```python
from build123d import *

# Parameters (mm, degrees)
SKETCH2_R           = 12.5
BOSS_EXTRUDE1_DEPTH = 6
SKETCH6_R           = 1.5
CUT_EXTRUDE1_DEPTH  = 15
SKETCH8_R           = 12.5
SKETCH8_R_2         = 10
BOSS_EXTRUDE2_DEPTH = 2
SKETCH9_R           = 2.5
CUT_EXTRUDE3_DEPTH  = 4


with BuildPart() as part:
    # Sketch2 → Boss-Extrude1 (new body)
    with BuildSketch(Plane.XY):
        Circle(SKETCH2_R)
    extrude(amount=BOSS_EXTRUDE1_DEPTH)

    # Sketch6 → Cut-Extrude1 (cut)
    with BuildSketch(Plane(origin=(0, 0, 0), x_dir=(-1, 0, 0), z_dir=(0, 0, -1))):
        with Locations((-5.488160471, -3.482828541)):
            Circle(SKETCH6_R)
        with Locations((-0.272137758, 6.494300658)):
            Circle(SKETCH6_R)
        with Locations((5.760298229, -3.011472117)):
            Circle(SKETCH6_R)
    extrude(amount=-CUT_EXTRUDE1_DEPTH, mode=Mode.SUBTRACT)

    # Sketch8 → Boss-Extrude2 (add)
    with BuildSketch(Plane(origin=(0, 0, 0), x_dir=(-1, 0, 0), z_dir=(0, 0, -1))):
        Circle(SKETCH8_R)
        Circle(SKETCH8_R_2, mode=Mode.SUBTRACT)
    extrude(amount=BOSS_EXTRUDE2_DEPTH)

    # Sketch9 → Cut-Extrude3 (cut)
    with BuildSketch(Plane(origin=(0, 0, 0), x_dir=(-1, 0, 0), z_dir=(0, 0, -1))):
        with Locations((-0.272137758, 6.494300658)):
            Circle(SKETCH9_R)
        with Locations((5.760298229, -3.011472117)):
            Circle(SKETCH9_R)
        with Locations((-5.488160471, -3.482828541)):
            Circle(SKETCH9_R)
    extrude(amount=-CUT_EXTRUDE3_DEPTH, mode=Mode.SUBTRACT)


solid = part.part
```
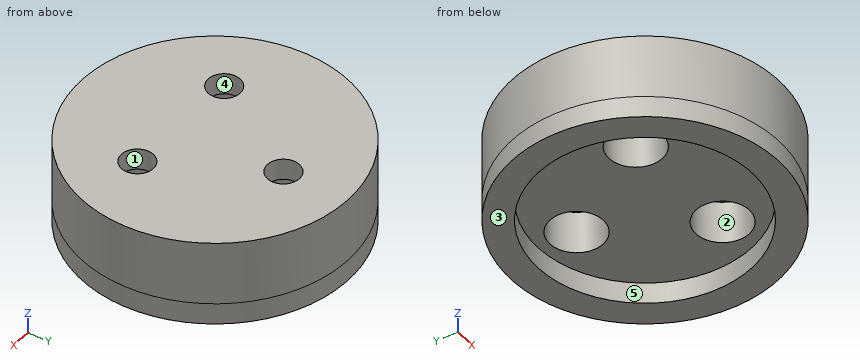
For this review, take the finished solid that the model builds, in its own axes (mm). Face numbers are marked on the shaded views. A direction names the side the tool comes from. Give positions to 0.01 mm unless a question says otherwise; leave off trailing zeros. Write each loop counter-clockwise with the first axis right and the second up, starting at its lowest first coordinate (ties: lowest second). Pieces come first, ordered by that corner, then holes. Notation, with made-up numbers: M -5.75,4 L 5.25,4 A14 cw 5.25,15 Z; hole C -11.75,88.25 d6. An arc over 180 degrees is marked long. Answer as a JSON object with one key per item and string values. Group by question number.
Item 1: For probe 1 along Y at (x, z) = (0, -1); probe 2 along X at (y, z) = (-2.5, 1); probe 3 along Z at (x, y) = (2.25, -1.75), list the stretches that pass through material, from the lowest coordinate up. Write a range as [from, to].
Item 2: Draft analysis for pull direction Y (two halves, no side actions). For the marked faces 3, 4 and 5, state which applies: +Y half, -Y half, draft (parallel to the pull), parting line (faces both ways), or undercut.
Item 3: For pin 1 Ø6 at (x, y) = (-3, 4.5) entering from -Z; pin 2 Ø4 at (x, y) = (0.27, 6.49) entering from -Z; pin 3 Ø2 at (x, z) = (-7, -1) entering from +Y, all flat-tipped, find the tip position at first contact; note any pin that passes through.
Item 4: Consider section D-D on x = 0. Write out the cut boundary in (y, z).
Item 5: Tool access review of the marked faces 1 and 2: name each direction out of +Z, -Z, +X, -X, +Y, -Y from which nothing blocks a thin tool from reaching the whole face with its end or side.
Item 6: Consider section C-C on z = -1.5. Write out the cut boundary in (x, y).
Item 7: Consider section A-A on x = -6.75. Write out the cut boundary in (y, z), plus the area to 3 significant figures.
Item 8: Consider section B-B on y = 0. Write out the cut boundary in (x, z), plus the area to 3 significant figures.
Check result:
{
 "1": {"probe 1": "y = [-12.5, -10], [10, 12.5]", "probe 2": "x = [-12.25, -8.21], [-3.31, 3.19], [7.79, 12.25]", "probe 3": "z = [0, 6]"},
 "2": {"face 3": "draft", "face 4": "undercut", "face 5": "undercut"},
 "3": {"pin 1": "stops at z = 0", "pin 2": "stops at z = 4", "pin 3": "stops at y = 10.97"},
 "4": {"outline": "M -12.5,-2 L -10,-2 L -10,0 L 4.01,0 L 4.01,4 L 5.02,4 L 5.02,6 L -12.5,6 Z; M 7.97,4 L 8.98,4 L 8.98,0 L 10,0 L 10,-2 L 12.5,-2 L 12.5,6 L 7.97,6 Z"},
 "5": {"face 1": "+Z, -Z", "face 2": "-Z"},
 "6": {"outline": "C 0,0 d25; hole C 0,0 d20"},
 "7": {"outline": "M -10.52,-2 L -7.38,-2 L -7.38,0 L -5.31,0 L -5.31,4 L -4.14,4 L -4.14,6 L -10.52,6 Z; M -1.88,4 L -0.72,4 L -0.72,0 L 7.38,0 L 7.38,-2 L 10.52,-2 L 10.52,6 L -1.88,6 Z", "area": "116 mm^2"},
 "8": {"outline": "M -12.5,-2 L -10,-2 L -10,0 L 10,0 L 10,-2 L 12.5,-2 L 12.5,6 L -12.5,6 Z", "area": "160 mm^2"}
}
